Read the model definition and answer for the solid it produces. Units are mm, in the model's axes. Coordinates: 2 decimals unless noted, no trailing zeros. Order: outer loops, then holes, each group sorted by start corner. A loop starts at its lowest first (then second) coordinate and runs counter-clockwise, first axis right, second up. Notation, with made-up numbers: M -14,44 L 7,44 A20 cw 7,68 Z; hole C 45.5,23 d3. An arc over 180 degrees is marked long. Write each question's results on one line, items separated by ' | '.
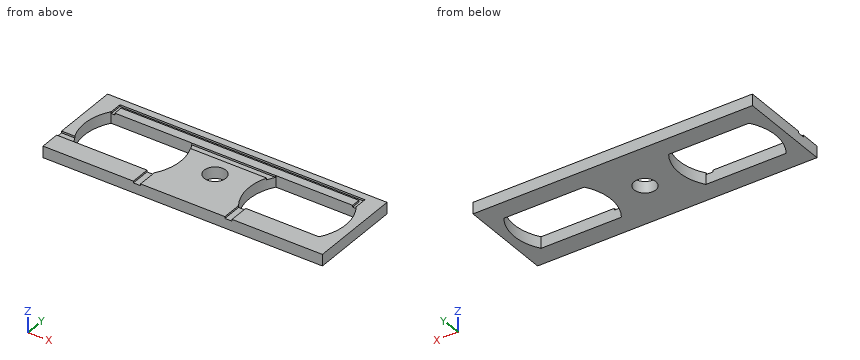
```python
from build123d import *

# Parameters (mm, degrees)
F0_W     = 39
F0_H     = 13
F1_DEPTH = 1.6
F2_W     = 1
F2_H     = 2.75
F3_DEPTH = 0.25
F4_R     = 1.5
F5_DEPTH = 1.601


with BuildPart() as f1:
    # F0 (on Top) → F1 (new body)
    with BuildSketch(Plane.XY):
        Rectangle(F0_W, F0_H)
        with BuildLine():
            ThreePointArc((-5.8875139198, 3.75), (-4.75, 0), (-5.8875139198, -3.75))
            Line((-5.8875139198, -3.75), (-17.1124860802, -3.75))
            ThreePointArc((-17.1124860802, -3.75), (-18.25, 0), (-17.1124860802, 3.75))
            Line((-17.1124860802, 3.75), (-5.8875139198, 3.75))
        make_face(mode=Mode.SUBTRACT)
        with BuildLine():
            ThreePointArc((5.8875139198, -3.75), (4.75, 0), (5.8875139198, 3.75))
            Line((5.8875139198, 3.75), (17.1124860802, 3.75))
            ThreePointArc((17.1124860802, 3.75), (18.25, 0), (17.1124860802, -3.75))
            Line((17.1124860802, -3.75), (5.8875139198, -3.75))
        make_face(mode=Mode.SUBTRACT)
    extrude(amount=F1_DEPTH)

    # F2 (on face) → F3 (cut)
    with BuildSketch(Plane.XY.offset(1.6)):
        Polygon((-17.0829144429, 5.5), (-17.0829144429, 3.75), (-16.5829144429, 3.75), (-16.5829144429, 5), (16.6124860802, 5), (16.6124860802, 3.75), (17.1124860802, 3.75), (17.1124860802, 5.5), align=None)
        with BuildLine():
            ThreePointArc((-5.8752075463, 3.7315157581), (-5.580137224, 3.2431041787), (-5.3273731959, 2.7315157581))
            Line((-5.3273731959, 2.7315157581), (5.3273731959, 2.7315157581))
            ThreePointArc((5.3273731959, 2.7315157581), (5.580137224, 3.2431041787), (5.8752075463, 3.7315157581))
            Line((5.8752075463, 3.7315157581), (-5.8752075463, 3.7315157581))
        make_face()
        with Locations((-6.3875139198, -5.125)):
            Rectangle(F2_W, F2_H)
        with BuildLine():
            Line((-19.5, -2.75), (-19.5, -3.75))
            Line((-19.5, -3.75), (-17.1124860802, -3.75))
            ThreePointArc((-17.1124860802, -3.75), (-17.4096399122, -3.2616952813), (-17.664414003, -2.75))
            Line((-17.664414003, -2.75), (-19.5, -2.75))
        make_face()
        with Locations((6.3875139198, -5.125)):
            Rectangle(F2_W, F2_H)
    extrude(amount=-F3_DEPTH, mode=Mode.SUBTRACT)

    # F4 (on face) → F5 (cut, through all)
    with BuildSketch(Plane.XY.offset(1.6)):
        Circle(F4_R)
    extrude(amount=-F5_DEPTH, mode=Mode.SUBTRACT)


solid = f1.part
```
(1) The part is cut by section D-D, the plane y = 3.25. Write down the section's boundary in (x, z).
Conclusion:
outline: M -19.5,0 L -17.42,0 L -17.42,1.6 L -19.5,1.6 Z; M -5.58,0 L 5.58,0 L 5.58,1.35 L -5.58,1.35 Z; M 17.42,0 L 19.5,0 L 19.5,1.6 L 17.42,1.6 Z
(2) Straight lines are drawn through the part: line 1 (Y direction, x = -7, z = 1.5); line 2 (Y direction, x = -3.5, z = 1.5); line 3 (Y direction, x = 0, z = 0.85). For each, find the intervals that lie inside material, in ascending order.
Conclusion:
line 1: -6.5 to -3.75, 3.75 to 5, 5.5 to 6.5 | line 2: -6.5 to 2.73, 3.73 to 5, 5.5 to 6.5 | line 3: -6.5 to -1.5, 1.5 to 6.5
(3) The part is cut by section A-A, the plane x = 0. Write down the section's boundary in (y, z).
Conclusion:
outline: M -6.5,0 L -1.5,0 L -1.5,1.6 L -6.5,1.6 Z; M 1.5,0 L 6.5,0 L 6.5,1.6 L 5.5,1.6 L 5.5,1.35 L 5,1.35 L 5,1.6 L 3.73,1.6 L 3.73,1.35 L 2.73,1.35 L 2.73,1.6 L 1.5,1.6 Z
(4) The part is cut by section C-C, the plane z = 0.6. Write down the section's boundary in (x, y), then the cut area to 3 significant figures.
Conclusion:
outline: M -19.5,-6.5 L 19.5,-6.5 L 19.5,6.5 L -19.5,6.5 Z; hole M -17.11,-3.75 L -5.89,-3.75 A6.75 ccw -5.89,3.75 L -17.11,3.75 A6.75 ccw Z; hole C 0,0 d3; hole M 5.89,-3.75 L 17.11,-3.75 A6.75 ccw 17.11,3.75 L 5.89,3.75 A6.75 ccw Z | area: 308 mm²
(5) The part is cut by section B-B, the plane y = 0. Write down the section's boundary in (x, z).
Conclusion:
outline: M -19.5,0 L -18.25,0 L -18.25,1.6 L -19.5,1.6 Z; M -4.75,0 L -1.5,0 L -1.5,1.6 L -4.75,1.6 Z; M 1.5,0 L 4.75,0 L 4.75,1.6 L 1.5,1.6 Z; M 18.25,0 L 19.5,0 L 19.5,1.6 L 18.25,1.6 Z
